Could you check a few things on this model? Use its own coordinates, in mm. A direction names the side the tool comes from. Round coordinates to 2 decimals unless told otherwise and drop trailing zeros. Write each loop counter-clockwise with the first axis right and the second up, starting at its lowest first coordinate (ties: lowest second). Pieces come first, ordered by that corner, then holes. Notation, with made-up numbers: (-4.75, -12.75) -> (8.25, -12.75) arc R18 cw to (8.25, 12.25) -> close; hole circle Ø11 at (7, 86). An arc over 180 degrees is marked (long way). Return JSON: item names as keys, results as strings.
from build123d import *

# Parameters (mm, degrees)
BOSS_EXTRUDE1_DEPTH = 1
SKETCH3_R           = 2.5
BOSS_EXTRUDE3_DEPTH = 7


with BuildPart() as part:
    # Sketch1 → Boss-Extrude1 (new body)
    with BuildSketch(Plane.XY):
        Polygon((0, 0), (86, 0), (86, 25), (65, 50), (0, 50), align=None)
    extrude(amount=BOSS_EXTRUDE1_DEPTH)

    # Sketch3 → Boss-Extrude3 (add)
    with BuildSketch(Plane.XY.offset(1)):
        with Locations((36.5, 11.5)):
            Circle(SKETCH3_R)
    extrude(amount=BOSS_EXTRUDE3_DEPTH)


solid = part.part
1) I want a section at A-A, the plane x = 36.5. Please give me the cut outline in (y, z).
Return value:
{"outline": "(0, 0) -> (50, 0) -> (50, 1) -> (14, 1) -> (14, 8) -> (9, 8) -> (9, 1) -> (0, 1) -> close"}
2) I want a section at C-C, the plane z = 5.75. Please give me the cut outline in (x, y), and give its area (3 significant figures).
Return value:
{"outline": "circle Ø5 at (36.5, 11.5)", "area": "19.6 mm²"}
3) I want a section at B-B, the plane y = 11.5. Please give me the cut outline in (x, z), and give its area (3 significant figures).
Return value:
{"outline": "(0, 0) -> (86, 0) -> (86, 1) -> (39, 1) -> (39, 8) -> (34, 8) -> (34, 1) -> (0, 1) -> close", "area": "121 mm²"}
4) I want a section at D-D, the plane y = 43. Please give me the cut outline in (x, z).
Return value:
{"outline": "(0, 0) -> (70.88, 0) -> (70.88, 1) -> (0, 1) -> close"}
5) Will these pins go through, and if not, where does the flat tip stop? pin 1 Ø4 at (x, z) = (10, 4) entering from -Y; pin 2 Ø3 at (x, y) = (44.5, 33) entering from +Z.
Return value:
{"pin 1": "through", "pin 2": "z = 1"}
6) If I drill on probe 1 along Z at (x, y) = (6.5, 5.5); probe 2 along X at (y, z) = (10, 1.75); probe 3 along X at (y, z) = (13.5, 2.5), over which ranges is the centre line in solid material (lowest first)? Write a range as [from, to].
Return value:
{"probe 1": "[0, 1]", "probe 2": "[34.5, 38.5]", "probe 3": "[35, 38]"}
7) For faces 1 (the face through (38.81, 10.54, 4.45)), 2 (the face through (75.647, 37.325, 0.493)), which set-ups out of +Z, -Z, +X, -X, +Y, -Y let a thin tool reach every point of the face, with its end or its side?
Return value:
{"face 1": "+Z", "face 2": "+Z, -Z, +X, +Y"}
